Here's how the part is built. I have some questions about the finished solid (model axes, mm). Round coordinates to 2 decimals unless told otherwise and drop trailing zeros. Loops run counter-clockwise (first coordinate to the right, second up) from the corner with the lowest first, then second, coordinate; pieces in that order, holes last. Notation, with made-up numbers: M -34,-32 L -24,-32 A21 cw -24,6 Z; hole C 83.25,15 d5. An arc over 180 degrees is marked long. Use a Markdown table: item, result.
from build123d import *

# Parameters (mm, degrees)
F0_W     = 38.1
F0_H     = 38.1
F1_DEPTH = 0.79375
F2_W     = 38.1
F2_H     = 38.1
F2_W_2   = 34.925
F2_H_2   = 34.925
F3_DEPTH = 5.08
F4_W     = 1.27
F4_H     = 4.4380559438
F5_DEPTH = 4.445
F4_H_2   = 7.9962998058
F4_H_3   = 5.8306083127
F4_H_4   = 4.9851979129
F4_H_5   = 9.1487001942
F6_DEPTH = 4.445
F4_R     = 1.27
F7_DEPTH = 0.396875
F8_DEPTH = 0.396875


# Not quite as in the source:
# - a feature names something its author has since deleted; it is built from what else it names


with BuildPart() as f1:
    # F0 (on Top) → F1 (new body)
    with BuildSketch(Plane.XY):
        with Locations((-0.0411514193, 3.4528287099)):
            Rectangle(F0_W, F0_H)
    extrude(amount=F1_DEPTH)

    # F2 (on face) → F3 (join)
    with BuildSketch(Plane.XY.offset(0.79375)):
        with Locations((-0.0411514193, 3.4528287099)):
            Rectangle(F2_W, F2_H)
        with Locations((-0.0411514193, 3.4528287099)):
            Rectangle(F2_W_2, F2_H_2, mode=Mode.SUBTRACT)
    extrude(amount=F3_DEPTH)

    # F4 (on face) → F5 (join)
    with BuildSketch(Plane.XY.offset(0.79375)):
        Polygon((3.4513485807, 6.6866285157), (-4.8036514193, 6.6866285157), (-4.8036514193, 5.4166285157), (1.5463485807, 5.4166285157), (1.5463485807, -3.0990629774), (11.0713485807, -3.0990629774), (11.0713485807, 5.1481691189), (11.0713485807, 5.4166285157), (11.0713485807, 8.1909499449), (9.8013485807, 8.1909499449), (9.8013485807, 6.6866285157), (4.7213485807, 6.6866285157), (4.7213485807, 13.2709499449), (12.3413485807, 13.2709499449), (12.3413485807, 14.2892440781), (12.3413485807, 15.8353287099), (9.8013485807, 15.8353287099), (9.8013485807, 14.2892440781), (4.7213485807, 14.2892440781), (4.7213485807, 15.8353287099), (3.4513485807, 15.8353287099), (1.5463485807, 15.8353287099), (0.2763485807, 15.8353287099), (0.2763485807, 11.7666285157), (1.5463485807, 11.7666285157), (3.4513485807, 11.7666285157), align=None)
        with Locations((16.7863485807, 5.971921973)):
            Rectangle(F4_W, F4_H)
    extrude(amount=F5_DEPTH)

    # F4 (on face) → F6 (join)
    with BuildSketch(Plane.XY.offset(0.79375)):
        Polygon((-11.1536514193, 15.8353287099), (-12.4236514193, 15.8353287099), (-12.4236514193, -14.0096712901), (-9.8836514193, -14.0096712901), (-9.8836514193, -0.9333714843), (-3.5336514193, -0.9333714843), (-3.5336514193, 0.3366285157), (-9.8836514193, 0.3366285157), (-9.8836514193, 6.2576471828), (-11.1536514193, 6.2576471828), align=None)
        with Locations((-4.1686514193, -10.0115213872)):
            Rectangle(F4_W, F4_H_2)
        with Locations((2.1813485807, -11.0943671338)):
            Rectangle(F4_W, F4_H_3)
        Polygon((7.8963485807, -8.1790629774), (7.8963485807, -14.0096712901), (17.4213485807, -14.0096712901), (17.4213485807, -8.1790629774), (16.1513485807, -8.1790629774), align=None)
        with Locations((16.7863485807, -5.686464021)):
            Rectangle(F4_W, F4_H_4)
        with Locations((-5.4386514193, 16.3409786128)):
            Rectangle(F4_W, F4_H_5)
    extrude(amount=F6_DEPTH)

    # F4 (on face) → F7 (cut)
    with BuildSketch(Plane.XY.offset(0.79375)):
        with Locations((-14.9636514193, -10.9013672918)):
            Circle(F4_R)
    extrude(amount=-F7_DEPTH, mode=Mode.SUBTRACT)

    # F4 (on face) → F8 (cut)
    with BuildSketch(Plane.XY.offset(0.79375)):
        with Locations((14.2290396616, 1.2073169928)):
            Circle(F4_R)
    extrude(amount=-F8_DEPTH, mode=Mode.SUBTRACT)


solid = f1.part
1. Imagine slicing it at B-B, the plane z = 4.05. State how many separate pieces and enclosed holes the cut face has, then the cut area to 3 significant figures.
Answer sheet:
| item | result |
|---|---|
| separate pieces | 2 |
| enclosed holes | 1 |
| area | 540 mm2 |
2. Imagine slicing it at A-A, the plane x = 9. Write out the boundary of the cut face in (y, z), then the cut area to 3 significant figures.
Answer sheet:
| item | result |
|---|---|
| outline | M -15.6,0 L 22.5,0 L 22.5,5.87 L 20.92,5.87 L 20.92,0.79 L 14.29,0.79 L 14.29,5.24 L 13.27,5.24 L 13.27,0.79 L 6.69,0.79 L 6.69,5.24 L -3.1,5.24 L -3.1,0.79 L -8.18,0.79 L -8.18,5.24 L -14.01,5.24 L -14.01,5.87 L -15.6,5.87 Z |
| area | 120 mm2 |
3. I need wall thicknesses on probe 1 along X at (y, z) = (-12, 1.5); probe 2 along Y at (x, z) = (-2.5, 2.3); probe 3 along X at (y, z) = (12, 3.4). Which ranges of each line are inside material? Lowest first, please. Write a range as from..to.
Answer sheet:
| item | result |
|---|---|
| probe 1 | -19.09..-17.5, -12.42..-9.88, -4.8..-3.53, 1.55..2.82, 7.9..19.01 |
| probe 2 | -15.6..-14.01, 5.42..6.69, 20.92..22.5 |
| probe 3 | -19.09..-17.5, -12.42..-11.15, -6.07..-4.8, 0.28..4.72, 17.42..19.01 |
4. For pin 1 Ø1 at (x, y) = (-1.5, 0.5) entering from +Z, with a flat end and sliding along its axis, tell me the tip position at first contact or that it passes through.
Answer sheet:
| item | result |
|---|---|
| pin 1 | z = 0.79 |
5. Imagine slicing it at C-C, the plane y = 19. Write out the boundary of the cut face in (x, z).
Answer sheet:
| item | result |
|---|---|
| outline | M -19.09,0 L 19.01,0 L 19.01,5.87 L 17.42,5.87 L 17.42,0.79 L -4.8,0.79 L -4.8,5.24 L -6.07,5.24 L -6.07,0.79 L -17.5,0.79 L -17.5,5.87 L -19.09,5.87 Z |
6. Imagine slicing it at D-D, the plane y = -9. Write out the boundary of the cut face in (x, z), then the cut area to 3 significant figures.
Answer sheet:
| item | result |
|---|---|
| outline | M -19.09,0 L 19.01,0 L 19.01,5.87 L 17.42,5.87 L 17.42,5.24 L 7.9,5.24 L 7.9,0.79 L 2.82,0.79 L 2.82,5.24 L 1.55,5.24 L 1.55,0.79 L -3.53,0.79 L -3.53,5.24 L -4.8,5.24 L -4.8,0.79 L -9.88,0.79 L -9.88,5.24 L -12.42,5.24 L -12.42,0.79 L -17.5,0.79 L -17.5,5.87 L -19.09,5.87 Z |
| area | 111 mm2 |
